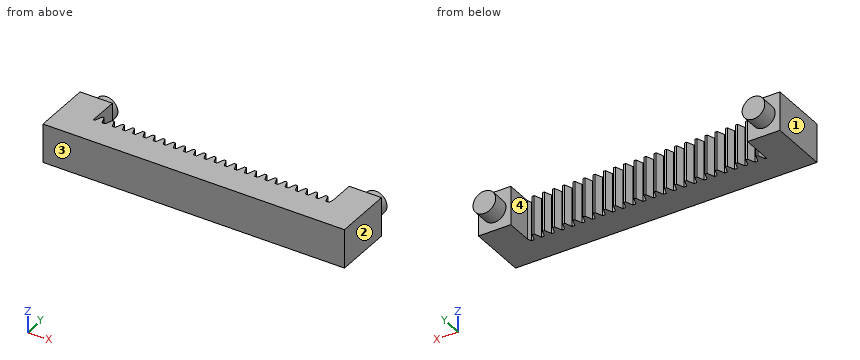
from build123d import *

# Parameters (mm, degrees)
BLANKSKE_W          = 73.1567043
BLANKSKE_H          = 11
BLANK_DEPTH         = 12
TOOTHCUTSIM_DEPTH   = 75.946003122
TEETHCUTS_COUNT     = 24
TEETHCUTS_PITCH     = 3.14159265
SKETCH1_W           = 12
SKETCH1_H           = 8.75
BOSS_EXTRUDE1_DEPTH = 10
SKETCH3_W           = 10
SKETCH3_H           = 8.75
BOSS_EXTRUDE2_DEPTH = 12
SKETCH4_W           = 10
SKETCH4_H           = 9.25
BOSS_EXTRUDE3_DEPTH = 12
SKETCH6_R           = 3.5
BOSS_EXTRUDE5_DEPTH = 5


with BuildPart() as part:
    # BlankSke → Blank (new body)
    with BuildSketch(Plane.XY):
        with Locations((36.57835215, 5.5)):
            Rectangle(BLANKSKE_W, BLANKSKE_H)
    extrude(amount=-BLANK_DEPTH)

    # TooCutSkeSim → ToothCutSim (cut, through all)
    with BuildSketch(Plane.XY):
        Polygon((0.44443537, 8.75), (-0.44443537, 8.75), (-1.272613241, 11.0254), (1.272613241, 11.0254), align=None)
    toothcutsim = extrude(amount=-TOOTHCUTSIM_DEPTH, mode=Mode.SUBTRACT)

    # TeethCuts: ToothCutSim ×24
    with Locations(*[(i * TEETHCUTS_PITCH, 0, 0) for i in range(1, TEETHCUTS_COUNT)]):
        add(toothcutsim, mode=Mode.SUBTRACT)

    # Sketch1 → Boss-Extrude1 (add)
    with BuildSketch(Plane.ZY):
        with Locations((-6, 4.375)):
            Rectangle(SKETCH1_W, SKETCH1_H)
    extrude(amount=BOSS_EXTRUDE1_DEPTH)

    # Sketch3 → Boss-Extrude2 (add, through all)
    with BuildSketch(Plane.XY):
        with Locations((78.1567043, 4.375)):
            Rectangle(SKETCH3_W, SKETCH3_H)
    extrude(amount=-BOSS_EXTRUDE2_DEPTH)

    # Sketch4 → Boss-Extrude3 (add, through all)
    with BuildSketch(Plane(origin=(0, 0, -12), x_dir=(-1, 0, 0), z_dir=(0, 0, -1))):
        with Locations((-78.1567043, 13.375)):
            Rectangle(SKETCH4_W, SKETCH4_H)
        with Locations((5, 13.375)):
            Rectangle(SKETCH4_W, SKETCH4_H)
    extrude(amount=-BOSS_EXTRUDE3_DEPTH)

    # Sketch6 → Boss-Extrude5 (add)
    with BuildSketch(Plane(origin=(0, 18, 0), x_dir=(1, 0, 0), z_dir=(0, 1, 0))):
        with Locations(Location((-5, 6, 0), (0, 0, 270))):
            Circle(SKETCH6_R)
        with Locations(Location((78.1567043, 6, 0), (0, 0, 270))):
            Circle(SKETCH6_R)
    extrude(amount=BOSS_EXTRUDE5_DEPTH)


solid = part.part
Work out the finished part from the listing and answer in its coordinate system (mm). Face numbers are marked on the shaded views. Round coordinates to 2 decimals unless told otherwise and drop trailing zeros. Order: outer loops, then holes, each group sorted by start corner. A loop starts at its lowest first (then second) coordinate and runs counter-clockwise, first axis right, second up. Notation, with made-up numbers: M 76,73 L 120,73 A33 ccw 120,107 Z; hole C 44,-31 d6. An arc over 180 degrees is marked long. Put each result on its own line as item: value. Start each with the question number.
Q1. Section A-A, the plane y = 13.25 is taken. Write down the section's boundary in (x, z), and give its area (3 significant figures).
Q2. Section C-C, the plane y = 21.5 is taken. Write down the section's boundary in (x, z), and give its area (3 significant figures).
Q3. Straight lines are drawn through the part: L1, parallel to X at y = 16.5, z = -9.25; L2, parallel to Y at x = 31, z = -4; L3, parallel to Y at x = 70.5, z = -6.5. For each, find the intervals that lie inside material, in ascending order. Write a range as [from, to].
Q4. Section B-B, the plane x = -5 is taken. Write down the section's boundary in (y, z), and give its area (3 significant figures).
Q5. For a pull along X with two mould halves and no side action, classify the marked faces 1, 2, 3 and 4 as pulls with the +X half, pulls with the -X half, needs draft (parallel to the pull), parting line crosses it, or undercut.
Q6. Flat-ended cylindrical pins translate along their axes: pin 1 (2 mm diameter, centred on x = 22.5, z = -7, fed in from +Y); pin 2 (5 mm diameter, centred on x = 15.5, z = -8.5, fed in from -Y); pin 3 (3 mm diameter, centred on y = 20, z = -10.5, fed in from -X). Find the tip coordinate at first contact, or state that the pin passes through.
Findings below:
1. outline: M -10,-12 L 0,-12 L 0,0 L -10,0 Z; M 73.16,-12 L 83.16,-12 L 83.16,0 L 73.16,0 Z
1. area: 240 mm^2
2. outline: C -5,-6 d7; C 78.16,-6 d7
2. area: 77.0 mm^2
3. L1: x = [-10, 0], [73.16, 83.16]
3. L2: y = [0, 8.75]
3. L3: y = [0, 11]
4. outline: M 0,-12 L 18,-12 L 18,-9.5 L 23,-9.5 L 23,-2.5 L 18,-2.5 L 18,0 L 0,0 Z
4. area: 251 mm^2
5. face 1: pulls with the -X half
5. face 2: pulls with the +X half
5. face 3: needs draft
5. face 4: undercut
6. pin 1: stops at y = 11
6. pin 2: stops at y = 0
6. pin 3: stops at x = -6.8
